Geometry: see drawing. Coordinates: mm, zero at the bounding-box minimum. A direction names the side the tool comes from. Give positions to 0.01 mm unless a question says otherwise; leave off trailing zeros. Loops run counter-clockwise (first coordinate to the right, second up) from the corner with the lowest first, then second, coordinate; pieces in that order, holes last. Notation, with made-up numbers: (15, 42.5) -> (69, 42.5) arc R25 ccw to (69, 60.5) -> close; hole circle Ø6 at (47, 57). An arc over 180 degrees is marked (long way). Use CSV: the item, a comma, the result in double quotes.
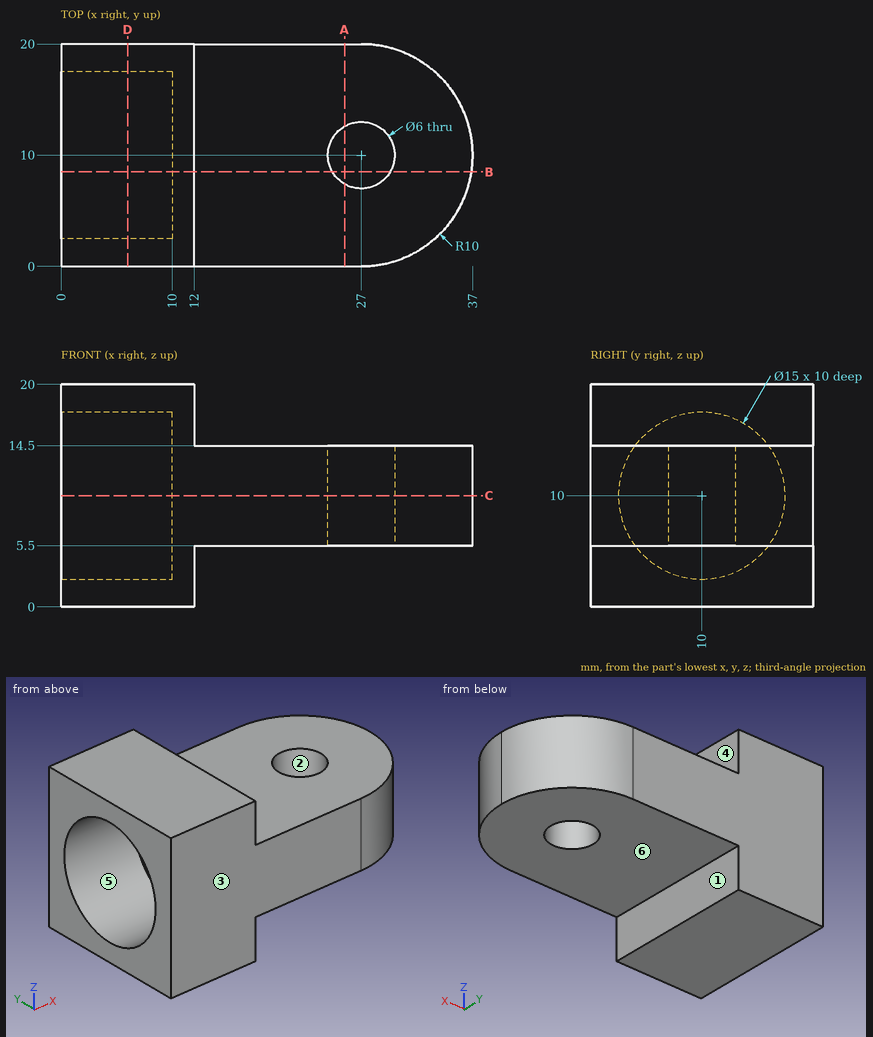
1) Section query D-D (x = 6). Return loops of the section in (y, z).
From the geometry:
outline,"(0, 0) -> (20, 0) -> (20, 20) -> (0, 20) -> close; hole circle Ø15 at (10, 10)"
2) Contact query for flat-ended pins moving along their axis: pin 1 (6 mm diameter, centred on y = 10, z = 18.5, fed in from +X); pin 2 (6 mm diameter, centred on y = 14.5, z = 7, fed in from +X); pin 3 (3 mm diameter, centred on x = 17, y = 10.5, fed in from -Z). Output: stop coordinate, or through.
From the geometry:
pin 1,"stops at x = 12"
pin 2,"stops at x = 36.89"
pin 3,"stops at z = 5.5"
3) Mould query, pull axis Y, two halves, no side actions, for the marked faces 1, 2 and 3. Classes: pulls with the +Y half, pulls with the -Y half, needs draft (parallel to the pull), parting line crosses it, or undercut.
From the geometry:
face 1,"needs draft"
face 2,"undercut"
face 3,"pulls with the -Y half"
4) Section query C-C (z = 10). Return loops of the section in (x, y), then the cut area to 3 significant figures.
From the geometry:
outline,"(0, 0) -> (27, 0) arc R10 ccw to (27, 20) -> (0, 20) -> (0, 17.5) -> (10, 17.5) -> (10, 2.5) -> (0, 2.5) -> close; hole circle Ø6 at (27, 10)"
area,"519 mm^2"
5) Section query B-B (y = 8.5). Return loops of the section in (x, z).
From the geometry:
outline,"(0, 0) -> (12, 0) -> (12, 5.5) -> (24.4, 5.5) -> (24.4, 14.5) -> (12, 14.5) -> (12, 20) -> (0, 20) -> (0, 17.35) -> (10, 17.35) -> (10, 2.65) -> (0, 2.65) -> close; (29.6, 5.5) -> (36.89, 5.5) -> (36.89, 14.5) -> (29.6, 14.5) -> close"
6) Section query A-A (x = 25.5). Return loops of the section in (y, z).
From the geometry:
outline,"(0, 5.5) -> (7.4, 5.5) -> (7.4, 14.5) -> (0, 14.5) -> close; (12.6, 5.5) -> (20, 5.5) -> (20, 14.5) -> (12.6, 14.5) -> close"
7) Reachability of the marked faces 4, 5 and 6 from +Z, -Z, +X, -X, +Y, -Y: full face, straight path, thin tool, end or side. Return the list, or none.
From the geometry:
face 4,"+Z, +X, +Y, -Y"
face 5,"-X"
face 6,"-Z, +X, +Y, -Y"
8) Ray query, line 1 (Y direction, x = 7.25, z = 10); line 2 (Y direction, x = 27, z = 8.5); line 3 (X direction, y = 8, z = 14.75). Return the intervals inside material, ascending.
From the geometry:
line 1,"y = 0 to 2.5, 17.5 to 20"
line 2,"y = 0 to 7, 13 to 20"
line 3,"x = 10 to 12"
